```python
from build123d import *

# Parameters (mm, degrees)
SKETCH1_R           = 25
BOSS_EXTRUDE1_DEPTH = 80
CUT_EXTRUDE1_DEPTH  = 80
SKETCH4_W           = 60
SKETCH4_H           = 145
CUT_EXTRUDE2_DEPTH  = 80
FILLET1_R           = 25
FILLET2_R           = 25
SKETCH5_R           = 12.5
BOSS_EXTRUDE2_DEPTH = 60


with BuildPart() as part:
    # Sketch1 → Boss-Extrude1 (new body)
    with BuildSketch(Plane.XY):
        with BuildLine():
            Line((-151.599161153, -67.5), (298.400838847, -67.5))
            Line((298.400838847, -67.5), (298.400838847, 67.5))
            Line((298.400838847, 67.5), (-151.599161153, 67.5))
            ThreePointArc((-151.599161153, 67.5), (-219.099161153, 0), (-151.599161153, -67.5))
        make_face()
        with Locations((-151.599161153, 0)):
            Circle(SKETCH1_R, mode=Mode.SUBTRACT)
    extrude(amount=BOSS_EXTRUDE1_DEPTH)

    # Sketch3 → Cut-Extrude1 (cut)
    with BuildSketch(Plane.XY.offset(80)):
        Polygon((298.400838847, 67.5), (-151.599161153, 67.5), (298.400838847, 47.5), align=None)
        Polygon((298.400838847, -67.5), (298.400838847, -47.5), (-151.599161153, -67.5), align=None)
    extrude(amount=-CUT_EXTRUDE1_DEPTH, mode=Mode.SUBTRACT)

    # Sketch4 → Cut-Extrude2 (cut)
    with BuildSketch(Plane(origin=(298.400838847, 0, 0), x_dir=(0, 0, -1), z_dir=(1, 0, 0))):
        with Locations((-40, 0)):
            Rectangle(SKETCH4_W, SKETCH4_H)
    extrude(amount=-CUT_EXTRUDE2_DEPTH, mode=Mode.SUBTRACT)

    # Fillet1
    fillet1_edges = [part.edges().sort_by_distance(p)[0] for p in [
        (218.400838847, -51.055555556, 40),
        (218.400838847, 51.055555556, 40),
    ]]
    fillet(fillet1_edges, radius=FILLET1_R)

    # Fillet2
    fillet2_edges = [part.edges().sort_by_distance(p)[0] for p in [
        (298.400838847, 47.5, 5),
        (298.400838847, -47.5, 5),
        (298.400838847, -47.5, 75),
        (298.400838847, 47.5, 75),
    ]]
    fillet(fillet2_edges, radius=FILLET2_R)

    # Sketch5 → Boss-Extrude2 (add)
    with BuildSketch(Plane.XY.offset(10)):
        with Locations(Location((259.510854188, 0, 0), (0, 0, 90))):
            Circle(SKETCH5_R)
    extrude(amount=BOSS_EXTRUDE2_DEPTH)


solid = part.part
```
The model under review builds one solid part; all positions refer to its coordinate system, in mm. A direction names the side the tool comes from. Round coordinates to 2 decimals unless told otherwise and drop trailing zeros. Order: outer loops, then holes, each group sorted by start corner. A loop starts at its lowest first (then second) coordinate and runs counter-clockwise, first axis right, second up. Notation, with made-up numbers: (72.5, 8.25) - (106.5, 8.25) arc R10 cw to (106.5, 16.25) - close; hole circle Ø5 at (51, 13). An arc over 180 degrees is marked (long way). Answer in a Markdown table with one row per item.
(1) Take a section at C-C on z = 42. Write out the cut boundary in (x, y).
Result set:
| item | result |
|---|---|
| outline | (-151.6, -67.5) - (194.51, -52.12) arc R25 ccw to (218.4, -27.14) - (218.4, 27.14) arc R25 ccw to (194.51, 52.12) - (-151.6, 67.5) arc R67.5 ccw to start; circle Ø25 at (259.51, 0); hole circle Ø50 at (-151.6, 0) |
(2) Mouldability with a two-part tool opening along X and no side actions: class faces 1 (the face through (247, -12, 10)), 2 (the face through (36, 1, 80)), 3 (the face through (291.65, -40.673, 4.93)) as released by +X, released by -X, zero draft, split by the parting line, or undercut.
Result set:
| item | result |
|---|---|
| face 1 | undercut |
| face 2 | zero draft |
| face 3 | released by +X |
(3) Clearance check with flat-ended pins moving along their axes: P1, Ø3, axis at x = 242, y = 52.5, coming from the +Z side; P2, Ø16.5, axis at y = 6.5, z = 41, coming from the +X side; P3, Ø1, axis at y = -44, z = 56, coming from the +X side; P4, Ø10, axis at x = -129, z = 46, coming from the -Y side. State where each tip first meets the part, or that it passes through.
Result set:
| item | result |
|---|---|
| P1 | passes through |
| P2 | stops at x = 272.01 |
| P3 | stops at x = 212.31 |
| P4 | stops at y = -66.72 |
(4) For line 1 (Z direction, x = 211, y = 51); line 2 (X direction, y = -18.5, z = 75); line 3 (Y direction, x = 259, z = 16), list the stretches that pass through material, from the lowest coordinate up. Write a range as from..to.
Result set:
| item | result |
|---|---|
| line 1 | z = 0..10, 70..80 |
| line 2 | x = -216.51..-168.41, -134.78..298.4 |
| line 3 | y = -12.49..12.49 |
(5) Take a section at B-B on z = 74.5. Write out the cut boundary in (x, y).
Result set:
| item | result |
|---|---|
| outline | (-151.6, -67.5) - (274.51, -48.56) arc R25 ccw to (298.4, -23.59) - (298.4, 23.59) arc R25 ccw to (274.51, 48.56) - (-151.6, 67.5) arc R67.5 ccw to start; hole circle Ø50 at (-151.6, 0) |
(6) Machinability: for faces 4 (the face through (211.281, 44.615, 40.42)), 5 (the face through (247, -12, 70)), 6 (the face through (-219.083, 1.484, 39.44)), 7 (the face through (211.281, -44.615, 39.58)), 8 (the face through (218.401, 0, 40)), which of the approach directions +Z, -Z, +X, -X, +Y, -Y give a long, thin tool a straight path to every point of the face, cutting with its end or side? Answer none if there is none.
Result set:
| item | result |
|---|---|
| face 4 | +X, +Y |
| face 5 | none |
| face 6 | +Z, -Z, -X |
| face 7 | +X, -Y |
| face 8 | +Y, -Y |
(7) Take a section at A-A on y = 0. Write out the cut boundary in (x, z).
Result set:
| item | result |
|---|---|
| outline | (-219.1, 0) - (-176.6, 0) - (-176.6, 80) - (-219.1, 80) - close; (-126.6, 0) - (298.4, 0) - (298.4, 10) - (272.01, 10) - (272.01, 70) - (298.4, 70) - (298.4, 80) - (-126.6, 80) - close; hole (218.4, 10) - (247.01, 10) - (247.01, 70) - (218.4, 70) - close |
(8) Take a section at D-D on x = -166. Write out the cut boundary in (y, z), plus the area to 3 significant figures.
Result set:
| item | result |
|---|---|
| outline | (-65.95, 0) - (-20.44, 0) - (-20.44, 80) - (-65.95, 80) - close; (20.44, 0) - (65.95, 0) - (65.95, 80) - (20.44, 80) - close |
| area | 7,280 mm2 |
